Autodesk Fusion 360 part; units mm, degrees
sketch "Sketch1" plane through (0, 0, 0) normal (0, 0, 1) x (1, 0, 0)
  circle A0 centre (0, 0) radius 3.175
  line L0 (-6.4231, 0) -> (-3.2116, -5.5626)
  line L1 (-3.2116, -5.5626) -> (3.2116, -5.5626)
  line L2 (3.2116, -5.5626) -> (6.4231, 0)
  line L3 (6.4231, 0) -> (3.2116, 5.5626)
  line L4 (3.2116, 5.5626) -> (-3.2116, 5.5626)
  line L5 (-3.2116, 5.5626) -> (-6.4231, 0)
  dimension "diameter" = 6.35
  dimension "hexwidth" = 11.1252
extrude "Extrude1" add sketch "Sketch1" along normal blind 5.7404
sketch "Sketch2" plane through (0, 0, 5.7404) normal (0, 0, 1) x (-1, 0, 0)
  circle A0 centre (0, 0) radius 3.175 construction
  line L0 (3.2116, -5.5626) -> (6.4231, 0) construction
  line L1 (6.4231, 0) -> (3.2116, 5.5626) construction
  line L2 (3.2116, 5.5626) -> (-3.2116, 5.5626) construction
  line L3 (-3.2116, 5.5626) -> (-6.4231, 0) construction
  line L4 (-6.4231, 0) -> (-3.2116, -5.5626) construction
  line L5 (-3.2116, -5.5626) -> (3.2116, -5.5626) construction
  circle A1 centre (0, 0) radius 5.5626
  circle A2 centre (0, 0) radius 30.9626
  dimension "hexcutoffset2" = 25.4
extrude "Extrude2" cut sketch "Sketch2" against normal blind 0.7366 draft -60
sketch "Sketch3" plane through (0, 0, 0) normal (0, 0, -1) x (1, 0, 0)
  circle A0 centre (0, 0) radius 3.175 construction
  line L0 (-6.4231, 0) -> (-3.2116, -5.5626) construction
  line L1 (-3.2116, -5.5626) -> (3.2116, -5.5626) construction
  line L2 (3.2116, -5.5626) -> (6.4231, 0) construction
  line L3 (6.4231, 0) -> (3.2116, 5.5626) construction
  line L4 (3.2116, 5.5626) -> (-3.2116, 5.5626) construction
  line L5 (-3.2116, 5.5626) -> (-6.4231, 0) construction
  circle A1 centre (0, 0) radius 5.5626
  circle A2 centre (0, 0) radius 30.9626
  dimension "hexcutoffset1" = 25.4
extrude "Extrude3" cut sketch "Sketch3" against normal blind 1.0414 draft -60
Read the model definition and answer for the solid it produces. Units are mm, in the model's axes. Round coordinates to 2 decimals unless told otherwise and drop trailing zeros. Write each loop counter-clockwise with the first axis right and the second up, starting at its lowest first coordinate (ties: lowest second). Pieces come first, ordered by that corner, then holes. Notation, with made-up numbers: (28, 85) - (83, 85) arc R9 ccw to (83, 99) - close; hole circle Ø7 at (71, 26). An arc over 180 degrees is marked (long way). Use CSV: the item, a comma, the result in double quotes.
Q1. Find section A-A, the plane z = 3.15. Write down the section's boundary in (x, y) (3 decimals), then the cut area to 3 significant figures.
Values:
outline,"(-6.423, 0) - (-3.212, -5.563) - (3.212, -5.563) - (6.423, 0) - (3.212, 5.563) - (-3.212, 5.563) - close; hole circle Ø6.35 at (0, 0)"
area,"75.5 mm²"
Q2. Determine the mould class of faces 1 (the conical face through (5.77, -0.01, 0.12)), 2 (the conical face through (-2.87, -5.01, 5.62)), 3 (the cylindrical face through (-0.69, 3.1, 2.83)) for opening direction Y: +Y half, -Y half, draft (parallel to the pull), parting line (faces both ways), or undercut.
Values:
face 1,"parting line"
face 2,"-Y half"
face 3,"undercut"
Q3. Straight lines are drawn through the part: line 1 along Y through (x, z) = (0, 3.6) (3 decimals); line 2 along X through (y, z) = (-0.5, 1.9); line 3 along Y through (x, z) = (0.75, 5.35). For each, find the intervals that lie inside material, in ascending order.
Values:
line 1,"y = -5.563 to -3.175, 3.175 to 5.563"
line 2,"x = -6.13 to -3.14, 3.14 to 6.13"
line 3,"y = -5.56 to -3.09, 3.09 to 5.56"
